from build123d import *

# Parameters (mm, degrees)
SKETCH1_W                    = 21.59
SKETCH1_H                    = 43.18
SKETCH1_R                    = 4.124999878
BOSS_EXTRUDE1_DEPTH          = 3.175
EDGE_FLANGE1_STRIP_W         = 19.05
EDGE_FLANGE1_STRIP_H         = 3.175
EDGE_FLANGE1_STRIP_CUT_DEPTH = 21.59
EDGE_FLANGE1_DEPTH           = 21.59
EDGE_FLANGE2_DEPTH           = 19.65452
EDGE_FLANGE2_START           = 3.175
EDGE_FLANGE2_FLAT_DEPTH      = 3.175
EDGE_FLANGE3_STRIP_W         = 15.900000204
EDGE_FLANGE3_STRIP_H         = 3.175
EDGE_FLANGE3_STRIP_CUT_DEPTH = 19.65452
EDGE_FLANGE3_DEPTH           = 19.65452
CUT_EXTRUDE2_REACH           = 97.152
SKETCH11_R                   = 2.55
FILLET1_R                    = 7.62


# Sheet-metal steps are written as plain solids
with BuildPart() as part:
    # Sketch1 → Boss-Extrude1 (new body)
    with BuildSketch(Plane.XY):
        with Locations((10.795, 0.048317484)):
            Rectangle(SKETCH1_W, SKETCH1_H)
        with Locations(Location((11.7183, 10.32174739, 0), (0, 0, 180))):
            Circle(SKETCH1_R, mode=Mode.SUBTRACT)
    extrude(amount=BOSS_EXTRUDE1_DEPTH)

    # Edge-Flange1: sheet metal written as solids
    # Edge-Flange1 strip (on a plane across the edge) → Edge-Flange1 strip cut (cut)
    with BuildSketch(Plane(origin=(21.59, -21.541682516, 0), x_dir=(0, 1, 0), z_dir=(-1, 0, 0))):
        with Locations((-6.35, -1.5875)):
            Rectangle(EDGE_FLANGE1_STRIP_W, EDGE_FLANGE1_STRIP_H)
    extrude(amount=EDGE_FLANGE1_STRIP_CUT_DEPTH, mode=Mode.SUBTRACT)

    # Edge-Flange1 section (on a plane across the edge) → Edge-Flange1 (add)
    with BuildSketch(Plane(origin=(21.59, -21.541682516, 0), x_dir=(0, 1, 0), z_dir=(-1, 0, 0))):
        with BuildLine():
            Line((-3.175, 3.175), (-3.175, 48.68672))
            Line((-3.175, 48.68672), (0, 48.68672))
            Line((0, 48.68672), (0, 3.175))
            ThreePointArc((0, 3.175), (0.92993597, 0.92993597), (3.175, 0))
            Line((3.175, 0), (3.175, -3.175))
            ThreePointArc((3.175, -3.175), (-1.315128061, -1.315128061), (-3.175, 3.175))
        make_face()
    extrude(amount=EDGE_FLANGE1_DEPTH)

    # Edge-Flange2: sheet metal written as solids
    # Edge-Flange2 bend section (on a plane across the edge) → Edge-Flange2 (add)
    with BuildSketch(Plane(origin=(-1.600000102, -24.716682516, -29.0322), x_dir=(1, 0, 0), z_dir=(0, 0, -1))):
        with BuildLine():
            Line((-3.175, 1.600000102), (0, 1.600000102))
            ThreePointArc((0, 1.600000102), (0.46862918, 0.46862918), (1.600000102, 0))
            Line((1.600000102, 0), (1.600000102, -3.175))
            ThreePointArc((1.600000102, -3.175), (-1.77643485, -1.77643485), (-3.175, 1.600000102))
        make_face()
    extrude(amount=EDGE_FLANGE2_DEPTH)

    # Edge-Flange2 profile (on flange) → Edge-Flange2 flat (add)
    with BuildSketch(Plane(origin=(-1.600000102, -24.716682516, 0), x_dir=(0, 0, -1), z_dir=(-1, 0, 0)).offset(EDGE_FLANGE2_START)):
        Polygon((29.0322, 28.10002), (29.0322, 19.3675), (29.0322, 1.600000102), (48.68672, 1.600000102), (48.68672, 28.10002), align=None)
    extrude(amount=-EDGE_FLANGE2_FLAT_DEPTH)

    # Edge-Flange3: sheet metal written as solids
    # Edge-Flange3 strip (on a plane across the edge) → Edge-Flange3 strip cut (cut)
    with BuildSketch(Plane(origin=(-1.600000102, -52.816702516, -29.0322), x_dir=(0, 1, 0), z_dir=(0, 0, -1))):
        with Locations((-3.175, -1.5875)):
            Rectangle(EDGE_FLANGE3_STRIP_W, EDGE_FLANGE3_STRIP_H)
    extrude(amount=EDGE_FLANGE3_STRIP_CUT_DEPTH, mode=Mode.SUBTRACT)

    # Edge-Flange3 section (on a plane across the edge) → Edge-Flange3 (add)
    with BuildSketch(Plane(origin=(-1.600000102, -52.816702516, -29.0322), x_dir=(0, 1, 0), z_dir=(0, 0, -1))):
        with BuildLine():
            Line((0, 1.600000102), (0, 35.364220102))
            Line((0, 35.364220102), (3.175, 35.364220102))
            Line((3.175, 35.364220102), (3.175, 1.600000102))
            ThreePointArc((3.175, 1.600000102), (3.64362918, 0.46862918), (4.775000102, 0))
            Line((4.775000102, 0), (4.775000102, -3.175))
            ThreePointArc((4.775000102, -3.175), (1.39856515, -1.77643485), (0, 1.600000102))
        make_face()
    extrude(amount=EDGE_FLANGE3_DEPTH)

    # Sketch11 → Cut-Extrude2 (cut, up to next)
    with BuildSketch(Plane.XZ.offset(52.816702516), mode=Mode.PRIVATE) as cut_extrude2_sk1:
        with Locations((24.17318, -38.85946)):
            Circle(SKETCH11_R)
    cut_extrude2_tool1 = extrude(cut_extrude2_sk1.sketch, amount=-CUT_EXTRUDE2_REACH, mode=Mode.PRIVATE) & part.part
    add(cut_extrude2_tool1.solids().sort_by_distance((24.17318, -52.816703, -38.85946))[0], mode=Mode.SUBTRACT)

    # Fillet1
    fillet1_edges = [part.edges().sort_by_distance(p)[0] for p in [
        (0, 21.638317484, 1.5875),
        (21.59, 21.638317484, 1.5875),
        (21.59, -23.129182516, -48.68672),
        (33.76422, -51.229202516, -29.0322),
        (33.76422, -51.229202516, -48.68672),
    ]]
    fillet(fillet1_edges, radius=FILLET1_R)


solid = part.part
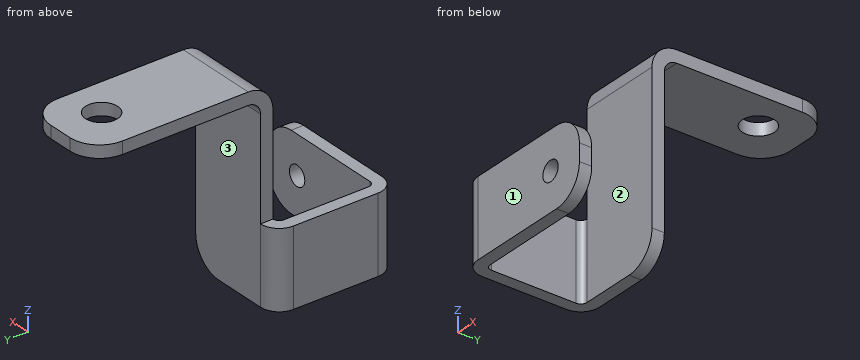
CAD build for the part. Positions are in the model's coordinates, mm. Face numbers are marked on the shaded views. A direction names the side the tool comes from. Round coordinates to 2 decimals unless told otherwise and drop trailing zeros. Order: outer loops, then holes, each group sorted by start corner. A loop starts at its lowest first (then second) coordinate and runs counter-clockwise, first axis right, second up. Notation, with made-up numbers: (64.25, -21) -> (96.25, -21) arc R7 cw to (96.25, -16) -> close; hole circle Ø5 at (-28, 32.25). An arc over 180 degrees is marked (long way). Write item = value, one per line. Start each with the question number.
(1) Cut at A-A, the plane y = 8.5. List the corners of the cut face in (x, z) (3 decimals), then the cut area to 3 significant figures.
(2) Cut at C-C, the plane z = -44.5. List the corners of the cut face in (x, y) (3 decimals).
(3) Pin check, flat tips, straight feed: P1, Ø1.5, axis at x = 18, z = -7.5, coming from the -Y side; P2, Ø7.5, axis at x = 11.72, y = 10.32, coming from the -Z side; P3, Ø6, axis at x = 24.17, z = -38.86, coming from the +Y side; P4, Ø6, axis at y = -37, z = -38, coming from the +X side. Stop position of each tip, or through.
(4) Cut at B-B, the plane x = 24.5. List the corners of the cut face in (y, z), then the cut area to 3 significant figures.
(5) Probe line 1 (Y direction, x = 16, z = -42); line 2 (Y direction, x = 5.5, z = -24); line 3 (Z direction, x = 18.5, y = -2.5) (3 decimals). List the from-to ranges inside material, lowest first. Write a range as [from, to].
(6) Which spindle directions (+Z, -Z, +X, -X, +Y, -Y) get a long thin tool onto all of the face, cutting with end or side? Do the marked faces 1, 2 and 3. Say none if no direction does.
(7) Cut at D-D, the plane y = -35.5. List the corners of the cut face in (x, z) (3 decimals), then the cut area to 3 significant figures.
Model answer:
q1.outline = (0, 0) -> (8.017, 0) -> (8.017, 3.175) -> (0, 3.175) -> close; (15.419, 0) -> (21.59, 0) -> (21.59, 3.175) -> (15.419, 3.175) -> close
q1.area = 45.0 mm2
q2.outline = (-4.775, -48.042) arc R4.775 ccw to (0, -52.817) -> (32.947, -52.817) -> (32.947, -49.642) -> (0, -49.642) arc R1.6 cw to (-1.6, -48.042) -> (-1.6, -26.317) arc R1.6 cw to (0, -24.717) -> (20.773, -24.717) -> (20.773, -21.542) -> (0, -21.542) arc R4.775 ccw to (-4.775, -26.317) -> close
q3.P1 = -24.72
q3.P2 = through
q3.P3 = -21.54
q3.P4 = -1.6
q4.outline = (-52.82, -48.69) -> (-49.64, -48.69) -> (-49.64, -41.39) -> (-52.82, -41.39) -> close; (-52.82, -36.33) -> (-49.64, -36.33) -> (-49.64, -29.03) -> (-52.82, -29.03) -> close
q4.area = 46.3 mm2
q5.line_1 = [-52.82, -49.64], [-24.72, -21.54]
q5.line_2 = [-24.72, -21.54]
q5.line_3 = [0, 3.175]
q6.face_1 = +Z, -Z, +X, -X, -Y
q6.face_2 = +Z, -Z, +X
q6.face_3 = -Z, +X, -X, +Y
q7.outline = (-4.775, -48.687) -> (-1.6, -48.687) -> (-1.6, -29.032) -> (-4.775, -29.032) -> close
q7.area = 62.4 mm2
